Autodesk Inventor part; units mm, degrees
ref_plane "YZ Plane" through (0, 0, 0) normal (1, 0, 0) x (0, 1, 0)
ref_plane "XZ Plane" through (0, 0, 0) normal (0, 1, 0) x (-1, 0, 0)
ref_plane "XY Plane" through (0, 0, 0) normal (0, 0, 1) x (1, 0, 0)
sketch "Sketch1" plane through (0, 0, 0) normal (0, 0, 1) x (1, 0, 0)
  circle A0 centre (-114.3, -4.6736) radius 2.1
  circle A1 centre (-114.3, -35.1536) radius 2.1
  circle A2 centre (0, -35.1536) radius 2.1
  circle A3 centre (0, -4.6736) radius 2.1
  line L0 (-114.9665, 7.2136) -> (0.6665, 7.2136)
  arc A4 (2.8956, 6.2995) -> (0.6665, 7.2136) centre (0.6665, 4.0386) ccw
  line L1 (2.8956, 6.2995) -> (13.6591, -4.3125)
  arc A5 (14.605, -6.5734) -> (13.6591, -4.3125) centre (11.43, -6.5734) ccw
  line L2 (14.605, -6.5734) -> (14.605, -33.2538)
  arc A6 (13.6591, -35.5147) -> (14.605, -33.2538) centre (11.43, -33.2538) ccw
  line L3 (13.6591, -35.5147) -> (2.8956, -46.1267)
  line L4 (0.6665, -47.0408) -> (-114.9665, -47.0408)
  arc A7 (0.6665, -47.0408) -> (2.8956, -46.1267) centre (0.6665, -43.8658) ccw
  arc A8 (-117.1956, -46.1267) -> (-114.9665, -47.0408) centre (-114.9665, -43.8658) ccw
  line L5 (-117.1956, -46.1267) -> (-127.9591, -35.5147)
  arc A9 (-128.905, -33.2538) -> (-127.9591, -35.5147) centre (-125.73, -33.2538) ccw
  line L6 (-128.905, -33.2538) -> (-128.905, -6.5734)
  arc A10 (-127.9591, -4.3125) -> (-128.905, -6.5734) centre (-125.73, -6.5734) ccw
  line L7 (-127.9591, -4.3125) -> (-117.1956, 6.2995)
  arc A11 (-114.9665, 7.2136) -> (-117.1956, 6.2995) centre (-114.9665, 4.0386) ccw
  point P0 (0, 0)
extrude "Extrusion1" add sketch "Sketch1" along normal blind 1
properties part number "Nameplatedrill"
The listing builds one solid part. Answer for the finished solid, in the listing's coordinates (mm). Give positions to 0.01 mm unless a question says otherwise; leave off trailing zeros. Write each loop counter-clockwise with the first axis right and the second up, starting at its lowest first coordinate (ties: lowest second). Pieces come first, ordered by that corner, then holes. Notation, with made-up numbers: (66, -27) -> (125, -27) arc R6 cw to (125, -20) -> close; hole circle Ø4 at (-38.5, 0). An arc over 180 degrees is marked (long way). Use a Markdown table: item, result.
(1) Determine the mould class of faces 1 (the cylindrical face through (-116.398, -4.766, 0.493)), 2 (the flat face through (8.4, -40.7, 0.5)), 3 (the flat face through (-122.65, 0.92, 0.49)) for opening direction Y: released by +Y, released by -Y, zero draft, split by the parting line, or undercut.
Return value:
| item | result |
|---|---|
| face 1 | undercut |
| face 2 | released by -Y |
| face 3 | released by +Y |
(2) Section A-A, the plane z = 0.85 is taken. Determine the outline of the cut face in (x, y) (1 decimal), then the cut area to 3 significant figures.
Return value:
| item | result |
|---|---|
| outline | (-128.9, -33.3) arc R3.2 ccw to (-128, -35.5) -> (-117.2, -46.1) arc R3.2 ccw to (-115, -47) -> (0.7, -47) arc R3.2 ccw to (2.9, -46.1) -> (13.7, -35.5) arc R3.2 ccw to (14.6, -33.3) -> (14.6, -6.6) arc R3.2 ccw to (13.7, -4.3) -> (2.9, 6.3) arc R3.2 ccw to (0.7, 7.2) -> (-115, 7.2) arc R3.2 ccw to (-117.2, 6.3) -> (-128, -4.3) arc R3.2 ccw to (-128.9, -6.6) -> close; hole circle Ø4.2 at (-114.3, -35.2); hole circle Ø4.2 at (-114.3, -4.7); hole circle Ø4.2 at (0, -35.2); hole circle Ø4.2 at (0, -4.7) |
| area | 7,410 mm2 |
(3) Find the intervals of material crossed by probe 1 along Y at (x, z) = (0, 0.75); probe 2 along X at (y, z) = (-37, 0.9); probe 3 along X at (y, z) = (5, 0.2), in increasing order. Write a range as from..to.
Return value:
| item | result |
|---|---|
| probe 1 | -47.04..-37.25, -33.05..-6.77, -2.57..7.21 |
| probe 2 | -126.45..-115.3, -113.3..-1, 1..12.15 |
| probe 3 | -118.51..4.21 |
(4) Section B-B, the plane y = -40 is taken. Determine the outline of the cut face in (x, z), then the cut area to 3 significant figures.
Return value:
| item | result |
|---|---|
| outline | (-123.41, 0) -> (9.11, 0) -> (9.11, 1) -> (-123.41, 1) -> close |
| area | 133 mm2 |
